```python
from build123d import *


with BuildPart() as part:
    # Sketch1 → Revolve3 (revolve)
    with BuildSketch(Plane.XY, mode=Mode.PRIVATE) as revolve3_sk:
        with BuildLine():
            Line((12.7, 0), (10.7, 0))
            Line((10.7, 0), (10.7, -3.884392891))
            Line((10.7, -3.884392891), (1.984375, -3.884392891))
            Line((1.984375, -3.884392891), (1.984375, -20.455909311))
            ThreePointArc((1.984375, -20.455909311), (2.995814611, -23.985925019), (0, -26.109392891))
            Line((0, -26.109392891), (0, 165.1))
            Line((0, 165.1), (7, 165.1))
            Line((7, 165.1), (7, 133.35))
            Line((7, 133.35), (7.62, 133.35))
            add(Edge.make_bspline(
                [(12.7, 101.6), (7.965904328, 117.119921913), (7.62, 133.35)],
                knots=[0, 0, 0, 1, 1, 1], degree=2))
            Line((12.7, 101.6), (12.7, 0))
        make_face()
    revolve(revolve3_sk.sketch.rotate(Axis((0, 165.1, 0), (0, -1, 0)), 90), axis=Axis((0, 165.1, 0), (0, -1, 0)))


solid = part.part
```
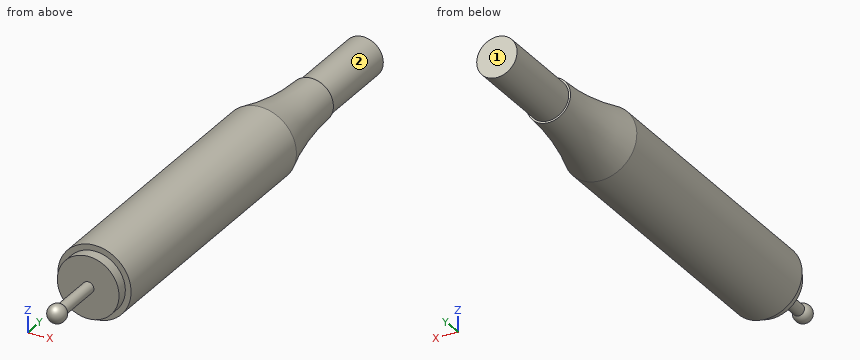
The listing builds one solid part. Answer for the finished solid, in the listing's coordinates (mm). Face numbers are marked on the shaded views. A direction names the side the tool comes from. Give positions to 0.01 mm unless a question says otherwise; leave off trailing zeros. Loops run counter-clockwise (first coordinate to the right, second up) from the corner with the lowest first, then second, coordinate; pieces in that order, holes last. Notation, with made-up numbers: (9, 58) - (52, 58) arc R31 ccw to (52, 91) - close; hole circle Ø8 at (39, 66). An arc over 180 degrees is marked (long way). Return JSON: item names as keys, results as strings. Group by question number.
1. Find section A-A (y = -2). Write down the section's boundary in (x, z).
2. Given pin 1 Ø8 at (y, z) = (97.5, 5.5) entering from +X; pin 2 Ø4 at (y, z) = (80, 9.5) entering from +X; pin 3 Ø12.5 at (x, z) = (1.5, -1.5) entering from -Y; pin 4 Ø3 at (x, z) = (-1, -2.5) entering from -Y, each flat-ended and moving along its own axis, determine where each tip first touches the part or whether it passes through.
3. Straight lines are drawn through the part: line 1 (Y direction, x = 4.5, z = 4.5); line 2 (Y direction, x = 1.25, z = -2); line 3 (X direction, y = 149.5, z = -0.5). For each, find the intervals that lie inside material, in ascending order. Write a range as [from, to].
4. Which of the six approach directions +Z, -Z, +X, -X, +Y, -Y give full straight-line access (tool end or side, diameter ignored) to the marked faces 1 and 2?
5. Find section B-B (y = 22.5). Write down the section's boundary in (x, z), then the cut area to 3 significant figures.
Verdict:
{
 "1": {"outline": "circle Ø21.4 at (0, 0)"},
 "2": {"pin 1": "stops at x = 12.61", "pin 2": "stops at x = 10.25", "pin 3": "stops at y = -26.11", "pin 4": "stops at y = -25.88"},
 "3": {"line 1": "y = [-3.88, 165.1]", "line 2": "y = [-25.06, -20.81], [-3.88, 165.1]", "line 3": "x = [-6.98, 6.98]"},
 "4": {"face 1": "+Z, -Z, +X, -X, +Y", "face 2": "+Y"},
 "5": {"outline": "circle Ø25.4 at (0, 0)", "area": "507 mm^2"}
}
